Can you work these out from the model? Positions are in its coordinate system, mm. Face numbers are marked on the shaded views. A direction names the side the tool comes from. Give positions to 0.01 mm unless a question says otherwise; leave off trailing zeros. Loops run counter-clockwise (first coordinate to the right, second up) from the corner with the lowest first, then second, coordinate; pieces in that order, holes last. Notation, with made-up numbers: (-14, 66.25) - (3, 66.25) arc R6 ccw to (3, 76.25) - close; hole circle Ø5 at (-16, 35.5). An arc over 180 degrees is marked (long way). Answer as a JSON object with one key per item and string values.
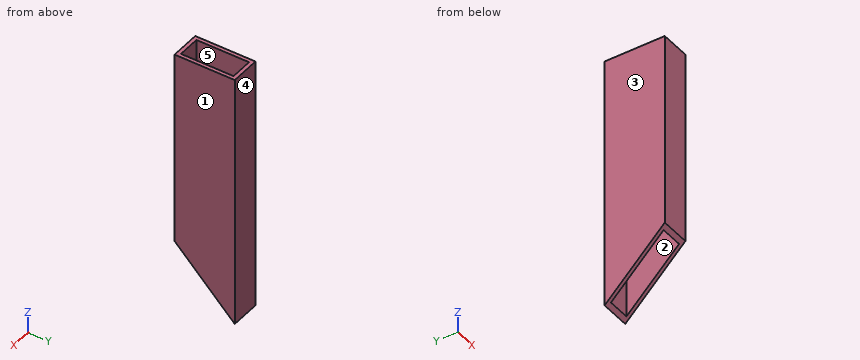
```python
from build123d import *

# Parameters (mm, degrees)
SKETCH1_W           = 25.4
SKETCH1_H           = 50.8
SKETCH1_W_2         = 19.05
SKETCH1_H_2         = 44.45
BOSS_EXTRUDE1_DEPTH = 215.9
CUT_EXTRUDE1_DEPTH  = 25.4


with BuildPart() as part:
    # Sketch1 → Boss-Extrude1 (new body)
    with BuildSketch(Plane.XY):
        with Locations((-12.7, 25.4)):
            Rectangle(SKETCH1_W, SKETCH1_H)
        with Locations((-12.7, 25.4)):
            Rectangle(SKETCH1_W_2, SKETCH1_H_2, mode=Mode.SUBTRACT)
    extrude(amount=BOSS_EXTRUDE1_DEPTH)

    # Sketch2 → Cut-Extrude1 (cut)
    with BuildSketch(Plane(origin=(0, 0, 0), x_dir=(0, 0, -1), z_dir=(1, 0, 0))):
        Polygon((0, 50.8), (-50.8, 0), (0, 0), align=None)
    extrude(amount=-CUT_EXTRUDE1_DEPTH, mode=Mode.SUBTRACT)


solid = part.part
```
1) Imagine slicing it at A-A on y = 6. Write out the boundary of the cut face in (x, z) (3 decimals).
Check sheet entries:
{"outline": "(-25.4, 44.8) - (-22.225, 44.8) - (-22.225, 215.9) - (-25.4, 215.9) - close; (-3.175, 44.8) - (0, 44.8) - (0, 215.9) - (-3.175, 215.9) - close"}
2) Imagine slicing it at C-C on z = 60. Write out the boundary of the cut face in (x, y) (3 decimals), and give its area (3 significant figures).
Check sheet entries:
{"outline": "(-25.4, 0) - (0, 0) - (0, 50.8) - (-25.4, 50.8) - close; hole (-22.225, 3.175) - (-3.175, 3.175) - (-3.175, 47.625) - (-22.225, 47.625) - close", "area": "444 mm2"}
3) Imagine slicing it at B-B on x = -11. Write out the boundary of the cut face in (y, z) (3 decimals), and give its area (3 significant figures).
Check sheet entries:
{"outline": "(0, 50.8) - (3.175, 47.625) - (3.175, 215.9) - (0, 215.9) - close; (47.625, 3.175) - (50.8, 0) - (50.8, 215.9) - (47.625, 215.9) - close", "area": "1,210 mm2"}
4) If we mould it in two halves opening along X, with no side actions, what happens to the marked faces 3, 4 and 5? For each: released by +X, released by -X, zero draft, split by the parting line, or undercut.
Check sheet entries:
{"face 3": "released by -X", "face 4": "zero draft", "face 5": "undercut"}
5) Imagine slicing it at D-D on z = 37. Write out the boundary of the cut face in (x, y) (3 decimals), and give its area (3 significant figures).
Check sheet entries:
{"outline": "(-25.4, 13.8) - (-22.225, 13.8) - (-22.225, 47.625) - (-3.175, 47.625) - (-3.175, 13.8) - (0, 13.8) - (0, 50.8) - (-25.4, 50.8) - close", "area": "295 mm2"}
6) Which directions (+Z, -Z, +X, -X, +Y, -Y) give clear straight access to the entire face, cutting with the end or side of a thin tool? Please do the marked faces 1 and 2.
Check sheet entries:
{"face 1": "+Z, -Z, +X, +Y, -Y", "face 2": "+Z, -Z"}
7) I'm going to push flat-ended pins straight in: P1, Ø5, axis at x = -21.5, y = 33, coming from the -Z side; P2, Ø1, axis at x = -8, z = 32.5, coming from the -Y side (3 decimals). Where does each tip first touch, or does it pass through?
Check sheet entries:
{"P1": "z = 15.41", "P2": "y = 47.625"}
8) I need wall thicknesses on L1, parallel to X at y = 32.5, z = 45 (3 decimals); L2, parallel to Y at x = -6, z = 169 (3 decimals); L3, parallel to Y at x = -18.25, z = 11 (3 decimals). Which ranges of each line are inside material? Lowest first, please.
Check sheet entries:
{"L1": "-25.4 to -22.225, -3.175 to 0", "L2": "0 to 3.175, 47.625 to 50.8", "L3": "47.625 to 50.8"}
